Autodesk Inventor part; units mm, degrees
ref_plane "YZ Plane" through (0, 0, 0) normal (1, 0, 0) x (0, 1, 0)
ref_plane "XZ Plane" through (0, 0, 0) normal (0, 1, 0) x (-1, 0, 0)
ref_plane "XY Plane" through (0, 0, 0) normal (0, 0, 1) x (1, 0, 0)
sketch "Sketch2" plane through (0, 0, 0) normal (1, 0, 0) x (0, 1, 0)
  line L0 (-25, 60) -> (-25, -60)
  line L1 (-25, -60) -> (25, -60)
  line L2 (-16, 60) -> (-16, -51)
  line L3 (-16, -51) -> (25, -51)
  line L4 (-16, 60) -> (-25, 60)
  line L5 (25, -60) -> (25, -51)
  point P0 (0, 0)
  point P1 (-25, 0)
  point P2 (0, -60)
  dimension "d1" = 120
  dimension "d2" = 50
  dimension "t" = 9
extrude "Extrusion1" add sketch "Sketch2" along normal mid plane 50
fillet "Fillet1" radius 9 1 edges at (0, -16, -51)
fillet "Fillet1" radius 18 1 edges at (0, -25, -60)
sketch "Sketch3" plane through (-25, -25, 60) normal (0, -1, 0) x (1, 0, 0)
  line L0 (50, 0) -> (0, 0)
  line L1 (0, -102) -> (0, 0)
  line L2 (50, 0) -> (50, -102)
  line L3 (5.5, -13) -> (5.5, -7) construction
  line L4 (8.8, -13) -> (8.8, -7)
  line L5 (2.2, -7) -> (2.2, -13)
  arc A0 (2.2, -13) -> (8.8, -13) centre (5.5, -13) ccw
  arc A1 (8.8, -7) -> (2.2, -7) centre (5.5, -7) ccw
  line L6 (25, -13) -> (25, -7) construction
  line L7 (28.3, -13) -> (28.3, -7)
  line L8 (21.7, -7) -> (21.7, -13)
  arc A2 (21.7, -13) -> (28.3, -13) centre (25, -13) ccw
  arc A3 (28.3, -7) -> (21.7, -7) centre (25, -7) ccw
  line L9 (44.5, -13) -> (44.5, -7) construction
  line L10 (47.8, -13) -> (47.8, -7)
  line L11 (41.2, -7) -> (41.2, -13)
  arc A4 (41.2, -13) -> (47.8, -13) centre (44.5, -13) ccw
  arc A5 (47.8, -7) -> (41.2, -7) centre (44.5, -7) ccw
  point P0 (25, -60)
  point P1 (5.5, -10)
  point P2 (25, -10)
  point P3 (44.5, -10)
  dimension "d8" = 10
  dimension "d9" = 5.5
  dimension "d10" = 5.5
  dimension "d11" = 39
  dimension "d12" = 19.5
  dimension "d29" = 3
  dimension "d30" = 6.6
  dimension "d31" = 6.6
sketch "Sketch4" plane through (-25, 25, -51) normal (0, 0, 1) x (1, 0, 0)
  line L0 (10, -7.5) -> (10, -25) construction
  line L1 (13.3, -7.5) -> (13.3, -25)
  line L2 (6.7, -25) -> (6.7, -7.5)
  arc A0 (13.3, -7.5) -> (6.7, -7.5) centre (10, -7.5) ccw
  arc A1 (6.7, -25) -> (13.3, -25) centre (10, -25) ccw
  line L3 (0, -32) -> (0, 0)
  line L4 (0, 0) -> (50, 0)
  line L5 (40, -7.5) -> (40, -25) construction
  line L6 (43.3, -7.5) -> (43.3, -25)
  line L7 (36.7, -25) -> (36.7, -7.5)
  arc A2 (43.3, -7.5) -> (36.7, -7.5) centre (40, -7.5) ccw
  arc A3 (36.7, -25) -> (43.3, -25) centre (40, -25) ccw
  point P0 (25, -25)
  point P1 (10, -16.25)
  point P2 (40, -16.25)
  dimension "d21" = 10
  dimension "d22" = 17.5
  dimension "d24" = 6.6
  dimension "d27" = 30
  dimension "d28" = 7.5
extrude "Extrusion2" cut sketch "Sketch4" along normal through all both and the other way through all
extrude "Extrusion3" cut sketch "Sketch3" along normal through all both and the other way through all
fillet "Fillet2" radius 5 4 edges at (-25, -20.5, 60) (25, -20.5, 60) (25, 25, -55.5) (-25, 25, -55.5)
equation "\"d6\" = t"
equation "\"d7\" = 2 * t"
properties part number "TL20240701-10200AT-005" material "SS400"
Verification items for the finished model (mm, model axes). A direction names the side the tool comes from. Coordinates: 2 decimals unless noted, no trailing zeros. Loops run counter-clockwise (first coordinate to the right, second up) from the corner with the lowest first, then second, coordinate; pieces in that order, holes last. Notation, with made-up numbers: (57, -16.75) - (69, -16.75) arc R19 ccw to (69, 19.25) - close; hole circle Ø10 at (32.25, 10.5). An arc over 180 degrees is marked (long way). Put each result on its own line as item: value.
Item 1: Set-up check for faces 4 (the face through (-14.9, -3.3, -55.6)), 5 (the face through (-23, 24, -55)), 6 (the face through (-19.4, -20.4, 43.7)): record each of +Z, -Z, +X, -X, +Y, -Y from which the full face is reachable in a straight line by a thin tool's end or side.
Conclusion:
face 4: +Z, -Z
face 5: +Z, -Z, -X, +Y
face 6: +Y, -Y
Item 2: Section check B-B (y = 5). Enter the section's corners in (x, z).
Conclusion:
outline: (-25, -60) - (-18.3, -60) - (-18.3, -51) - (-25, -51) - close; (-11.7, -60) - (11.7, -60) - (11.7, -51) - (-11.7, -51) - close; (18.3, -60) - (25, -60) - (25, -51) - (18.3, -51) - close
Item 3: Section check D-D (x = 6). Enter the section's corners in (y, z).
Conclusion:
outline: (-25, -42) arc R18 ccw to (-7, -60) - (25, -60) - (25, -51) - (-7, -51) arc R9 cw to (-16, -42) - (-16, 60) - (-25, 60) - close
Item 4: Scan lines: line 1 along X through (y, z) = (-19.5, 50.5); line 2 along X through (y, z) = (4, -52); line 3 along Y through (x, z) = (6.5, -5). Record each from-to range of solid material in increasing order.
Conclusion:
line 1: x = -25 to -22.8, -16.2 to -3.3, 3.3 to 16.2, 22.8 to 25
line 2: x = -25 to -18.3, -11.7 to 11.7, 18.3 to 25
line 3: y = -25 to -16
Item 5: Gauge pin test, flat ends, axial feed: pin 1 Ø1 at (x, z) = (-7, 46) entering from +Y; pin 2 Ø9.5 at (x, y) = (9.5, 3) entering from +Z. Record the tip position at first contact, or that the pin passes through.
Conclusion:
pin 1: stops at y = -16
pin 2: stops at z = -51
Item 6: Draft check along Z on faces 1 (the face through (24, -21, 58)), 2 (the face through (25, -18, -11)), 3 (the face through (-16.2, -20, 50)). Enter one of: pulls with the +Z half, pulls with the -Z half, needs draft (parallel to the pull), parting line crosses it, or undercut.
Conclusion:
face 1: pulls with the +Z half
face 2: needs draft
face 3: undercut
Item 7: Section check C-C (z = -22). Enter the section's corners in (x, y).
Conclusion:
outline: (-25, -25) - (25, -25) - (25, -16) - (-25, -16) - close
Item 8: Section check A-A (x = 0). Enter the section's corners in (y, z), then the cut area to 3 significant figures.
Conclusion:
outline: (-25, -42) arc R18 ccw to (-7, -60) - (25, -60) - (25, -51) - (-7, -51) arc R9 cw to (-16, -42) - (-16, 43.7) - (-25, 43.7) - close; (-25, 56.3) - (-16, 56.3) - (-16, 60) - (-25, 60) - close
area: 1,280 mm2
